from build123d import *

# Parameters (mm, degrees)
F0_W     = 544
F0_H     = 50
F1_DEPTH = 6
F2_W     = 544
F2_H     = 6
F3_DEPTH = 44
F4_R     = 9
F5_DEPTH = 25


with BuildPart() as f1:
    # F0 (on Front) → F1 (new body)
    with BuildSketch(Plane.XZ):
        with Locations((272, 25)):
            Rectangle(F0_W, F0_H)
    extrude(amount=F1_DEPTH)

    # F2 (on face) → F3 (join)
    with BuildSketch(Plane.XZ.offset(6)):
        with Locations((272, 47)):
            Rectangle(F2_W, F2_H)
    extrude(amount=F3_DEPTH)

    # F4 (on face) → F5 (cut)
    with BuildSketch(Plane(origin=(0, 0, 0), x_dir=(-1, 0, 0), z_dir=(0, 1, 0))):
        with Locations((-516, 22)):
            Circle(F4_R)
        with Locations((-28, 22)):
            Circle(F4_R)
    extrude(amount=-F5_DEPTH, mode=Mode.SUBTRACT)


solid = f1.part
The listing builds one solid part. Answer for the finished solid, in the listing's coordinates (mm). A direction names the side the tool comes from. Coordinates: 2 decimals unless noted, no trailing zeros. Order: outer loops, then holes, each group sorted by start corner. A loop starts at its lowest first (then second) coordinate and runs counter-clockwise, first axis right, second up.
Q1. A cutting plane is placed at C-C, the plane x = 364.5. Write down the section's boundary in (y, z), and give its area (3 significant figures).
Q2. A cutting plane is placed at D-D, the plane y = -38. Write down the section's boundary in (x, z).
Q3. A cutting plane is placed at A-A, the plane z = 22. Write down the section's boundary in (x, y).
Q4. Consider line 1 (Z direction, x = 516, y = -2.05); line 2 (Z direction, x = 319.5, y = -28); line 3 (Y direction, x = 381, z = 21.5). Determine where each line is inside the solid, lowest interval first.
Q5. A cutting plane is placed at B-B, the plane x = 28. Write down the section's boundary in (y, z).
Q6. Given P1, Ø2, axis at x = 434.5, z = 43.5, coming from the +Y side; P2, Ø2, axis at x = 323.5, y = -24.5, coming from the -Z side; P3, Ø11, axis at x = 28, z = 22, coming from the -Y side; P4, Ø12, axis at x = 281, z = 13.5, coming from the -Y side, each flat-ended and moving along its own axis, determine where each tip first touches the part or whether it passes through.
Q7. Which of the six approach directions +Z, -Z, +X, -X, +Y, -Y give full straight-line access (tool end or side, diameter ignored) to faces 4 (the face through (268, -28, 44)), 5 (the face through (268, 0, 25))?
Q8. For a pull along X with two mould halves and no side action, classify faces 1 (the face through (507.416, -2.958, 24.703)), 2 (the face through (544, -5, 34)), 3 (the face through (268, -25, 50)) as pulls with the +X half, pulls with the -X half, needs draft (parallel to the pull), parting line crosses it, or undercut.
Answers follow:
1. outline: (-50, 44) - (-6, 44) - (-6, 0) - (0, 0) - (0, 50) - (-50, 50) - close
1. area: 564 mm2
2. outline: (0, 44) - (544, 44) - (544, 50) - (0, 50) - close
3. outline: (0, -6) - (19, -6) - (19, 0) - (0, 0) - close; (37, -6) - (507, -6) - (507, 0) - (37, 0) - close; (525, -6) - (544, -6) - (544, 0) - (525, 0) - close
4. line 1: z = 0 to 13, 31 to 50
4. line 2: z = 44 to 50
4. line 3: y = -6 to 0
5. outline: (-50, 44) - (-6, 44) - (-6, 31) - (0, 31) - (0, 50) - (-50, 50) - close; (-6, 0) - (0, 0) - (0, 13) - (-6, 13) - close
6. P1: stops at y = 0
6. P2: stops at z = 44
6. P3: passes through
6. P4: stops at y = -6
7. face 4: -Z, +X, -X, -Y
7. face 5: +Z, -Z, +X, -X, +Y
8. face 1: undercut
8. face 2: pulls with the +X half
8. face 3: needs draft
